Source: CAD feature listing. Evaluate the final solid. Frame: model axes, mm. A direction names the side the tool comes from. Round coordinates to 2 decimals unless told otherwise and drop trailing zeros. Order: outer loops, then holes, each group sorted by start corner. A loop starts at its lowest first (then second) coordinate and runs counter-clockwise, first axis right, second up. Notation, with made-up numbers: M 22,-39 L 48,-39 A17 cw 48,-27 Z; hole C 66,69.5 d5. An arc over 180 degrees is marked long. Use one line per item in the form item = value. Start each with the question number.
Q1. Pull-direction query (Z, two-part tool) for faces 3 (the flat face through (-17.16, -4.93, -5.29)), 4 (the flat face through (7, 0, -7)); classes: pulls with the +Z half, pulls with the -Z half, needs draft (parallel to the pull), parting line crosses it, or undercut.
Q2. Section A-A (x = 0). Give the number of separate pieces and of enclosed holes in the cut face, plus the area to 3 significant figures.
Q3. Section B-B (y = -6). Return the cut outline in (x, z), plus the area to 3 significant figures.
Q4. Reachability of faces 1 (the cylindrical face through (-21.185, -4.93, -18.655)), 2 (the flat face through (7, -10, -7)) from +Z, -Z, +X, -X, +Y, -Y: full face, straight path, thin tool, end or side. Return the list, or none.
Q5. Material intervals for probe 1 along Z at (x, y) = (0, -6.5); probe 2 along Z at (x, y) = (9, -3); probe 3 along X at (y, z) = (-8, 11), sorted ascending.
Q6. Contact query for a flat-ended pin moving along its axis: pin 1 (1.5 mm diameter, centred on y = -1.5, z = -3, fed in from -X). Output: stop coordinate, or through.
from build123d import *

# Parameters (mm, degrees)
F0_R     = 7.5
F1_DEPTH = 10
F2_R     = 4.99999


# Not quite as in the source:
# - a fillet or chamfer is up to 0.001 mm smaller than in the source, because OpenCascade refuses the exact size


with BuildPart() as f1:
    # F0 (on Front) → F1 (new body)
    with BuildSketch(Plane.XZ):
        with BuildLine():
            ThreePointArc((-3.3902032697, 39.8560725836), (-27.0591192504, -29.4585143107), (40, 0))
            ThreePointArc((40, 0), (29.6647939484, 26.83281573), (4, 39.7994974843))
            ThreePointArc((4, 39.7994974843), (0.3062077702, 39.9988279428), (-3.3902032697, 39.8560725836))
        make_face()
        with BuildLine():
            ThreePointArc((-29.6388118521, -4.6412101868), (-25.7834406394, 15.3366941937), (-10.0682439236, 28.2600506775))
            ThreePointArc((-10.0682439236, 28.2600506775), (-5.5083812132, 27.6360062099), (-3.3902032697, 23.5500422312))
            Line((-3.3902032697, 23.5500422312), (-3.3902032697, 12.0314804488))
            ThreePointArc((-3.3902032697, 12.0314804488), (0.3191719091, 12.4959245073), (4, 11.8427192823))
            Line((4, 11.8427192823), (4, 23.3238075794))
            ThreePointArc((4, 23.3238075794), (6.1715728753, 27.446913205), (10.8, 27.9885690953))
            ThreePointArc((10.8, 27.9885690953), (26.1736871016, 14.6607674939), (29.5080437608, -5.4106703294))
            ThreePointArc((29.5080437608, -5.4106703294), (26.6876740435, -9.0476050406), (22.0900364673, -8.8390189601))
            Line((22.0900364673, -8.8390189601), (12.1146693487, -3.0797380689))
            ThreePointArc((12.1146693487, -3.0797380689), (10.6622021125, -6.5243732351), (8.2560957484, -9.3854612563))
            Line((8.2560957484, -9.3854612563), (18.1990098767, -15.1260054048))
            ThreePointArc((18.1990098767, -15.1260054048), (20.6839376534, -19.0681954938), (18.8388118521, -23.3473589085))
            ThreePointArc((18.8388118521, -23.3473589085), (-0.3902464621, -29.9974616876), (-19.4397998371, -22.8493803481))
            ThreePointArc((-19.4397998371, -22.8493803481), (-21.1792928303, -18.5884011693), (-18.6998331976, -14.7110232712))
            Line((-18.6998331976, -14.7110232712), (-8.724466079, -8.95174238))
            ThreePointArc((-8.724466079, -8.95174238), (-10.9813740217, -5.9715512722), (-12.2560957484, -2.457258026))
            Line((-12.2560957484, -2.457258026), (-22.1990098767, -8.1978021746))
            ThreePointArc((-22.1990098767, -8.1978021746), (-26.8555105286, -8.3787177112), (-29.6388118521, -4.6412101868))
        make_face(mode=Mode.SUBTRACT)
        with BuildLine():
            ThreePointArc((4, 11.8427192823), (0.3191719091, 12.4959245073), (-3.3902032697, 12.0314804488))
            ThreePointArc((-3.3902032697, 12.0314804488), (-10.6622021125, 6.5243732351), (-12.2560957484, -2.457258026))
            ThreePointArc((-12.2560957484, -2.457258026), (-10.9813740217, -5.9715512722), (-8.724466079, -8.95174238))
            ThreePointArc((-8.724466079, -8.95174238), (-0.3191719091, -12.4959245073), (8.2560957484, -9.3854612563))
            ThreePointArc((8.2560957484, -9.3854612563), (10.6622021125, -6.5243732351), (12.1146693487, -3.0797380689))
            ThreePointArc((12.1146693487, -3.0797380689), (12.4032932493, -1.5518751789), (12.5, 0))
            ThreePointArc((12.5, 0), (10.1550480058, 7.2886898686), (4, 11.8427192823))
        make_face()
        Circle(F0_R, mode=Mode.SUBTRACT)
    extrude(amount=F1_DEPTH)

    # F2 (radius 5 in the source; OpenCascade refuses exactly that, so slightly less here)
    f2_edges = [f1.edges().sort_by_distance(p)[0] for p in [
        (-40, -10, 0),
        (-40, 0, 0),
    ]]
    fillet(f2_edges, radius=F2_R)


solid = f1.part
Results list:
q1.face_3 = undercut
q1.face_4 = needs draft
q2.separate_pieces = 3
q2.enclosed_holes = 0
q2.area = 454 mm2
q3.outline = C 0,0 d79.8; hole M -29.64,-4.64 A5 ccw -22.2,-8.2 L -12.26,-2.46 A12.5 cw -3.39,12.03 L -3.39,23.55 A5 ccw -10.07,28.26 A30 ccw Z; hole M -19.44,-22.85 A30 ccw 18.84,-23.35 A5 ccw 18.2,-15.13 L 8.26,-9.39 A12.5 cw -8.72,-8.95 L -18.7,-14.71 A5 ccw Z; hole C 0,0 d15; hole M 4,11.84 A12.5 cw 12.11,-3.08 L 22.09,-8.84 A5 ccw 29.51,-5.41 A30 ccw 10.8,27.99 A5 ccw 4,23.32 Z
q3.area = 2,940 mm2
q4.face_1 = +Y, -Y
q4.face_2 = +Z, -Z, +X, -X, -Y
q5.probe_1 = -39.77 to -30, -12.5 to -7.5, 7.5 to 39.77
q5.probe_2 = -38.55 to -28.62, -9.81 to 8.67, 28.32 to 38.55
q5.probe_3 = -37.42 to -27.91, -5.94 to 5.94, 27.91 to 37.42
q6.pin_1 = -39.06
